from build123d import *

# Parameters (mm, degrees)
SKETCH_1_W          = 15
SKETCH_1_H          = 15
SKETCH_1_W_2        = 12
SKETCH_1_H_2        = 12
EXTRUDE_1_DEPTH     = 600
SKETCH_2_R          = 2.7
CUT_EXTRUDE_1_DEPTH = 25
SKETCH_3_R          = 2.25
CUT_EXTRUDE_2_DEPTH = 25
SKETCH_4_R          = 2.7
CUT_EXTRUDE_3_DEPTH = 20
SKETCH_5_R          = 5
CUT_EXTRUDE_4_DEPTH = 10
SKETCH_6_R          = 5
CUT_EXTRUDE_5_DEPTH = 10


with BuildPart() as part:
    # ｽｹｯﾁ1 → ﾎﾞｽ - 押し出し1 (new body)
    with BuildSketch(Plane.XY):
        Rectangle(SKETCH_1_W, SKETCH_1_H)
        Rectangle(SKETCH_1_W_2, SKETCH_1_H_2, mode=Mode.SUBTRACT)
    extrude(amount=EXTRUDE_1_DEPTH)

    # ｽｹｯﾁ2 → ｶｯﾄ - 押し出し1 (cut)
    with BuildSketch(Plane(origin=(7.5, 0, 0), x_dir=(0, 0, -1), z_dir=(1, 0, 0))):
        with Locations((-592.5, 0)):
            Circle(SKETCH_2_R)
        with Locations((-7.5, 0)):
            Circle(SKETCH_2_R)
    extrude(amount=-CUT_EXTRUDE_1_DEPTH, mode=Mode.SUBTRACT)

    # ｽｹｯﾁ3 → ｶｯﾄ - 押し出し2 (cut)
    with BuildSketch(Plane(origin=(0, 7.5, 0), x_dir=(1, 0, 0), z_dir=(0, 1, 0))):
        with Locations((0, -22.5)):
            Circle(SKETCH_3_R)
        with Locations((0, -577.5)):
            Circle(SKETCH_3_R)
        with Locations((0, -248.5)):
            Circle(SKETCH_3_R)
        with Locations((0, -351.5)):
            Circle(SKETCH_3_R)
    extrude(amount=-CUT_EXTRUDE_2_DEPTH, mode=Mode.SUBTRACT)

    # ｽｹｯﾁ4 → ｶｯﾄ - 押し出し3 (cut)
    with BuildSketch(Plane(origin=(7.5, 0, 0), x_dir=(0, 0, -1), z_dir=(1, 0, 0))):
        with Locations((-366.5, 0)):
            Circle(SKETCH_4_R)
        with Locations((-233.5, 0)):
            Circle(SKETCH_4_R)
    extrude(amount=-CUT_EXTRUDE_3_DEPTH, mode=Mode.SUBTRACT)

    # ｽｹｯﾁ5 → ｶｯﾄ - 押し出し4 (cut)
    with BuildSketch(Plane(origin=(7.5, 0, 0), x_dir=(0, 0, -1), z_dir=(1, 0, 0))):
        with Locations((-592.5, 0)):
            Circle(SKETCH_5_R)
        with Locations((-366.5, 0)):
            Circle(SKETCH_5_R)
        with Locations((-233.5, 0)):
            Circle(SKETCH_5_R)
        with Locations((-7.5, 0)):
            Circle(SKETCH_5_R)
    extrude(amount=-CUT_EXTRUDE_4_DEPTH, mode=Mode.SUBTRACT)

    # ｽｹｯﾁ6 → ｶｯﾄ - 押し出し5 (cut)
    with BuildSketch(Plane(origin=(0, -7.5, 0), x_dir=(-1, 0, 0), z_dir=(0, -1, 0))):
        with Locations((0, -577.5)):
            Circle(SKETCH_6_R)
        with Locations((0, -22.5)):
            Circle(SKETCH_6_R)
        with Locations((0, -248.5)):
            Circle(SKETCH_6_R)
        with Locations((0, -351.5)):
            Circle(SKETCH_6_R)
    extrude(amount=-CUT_EXTRUDE_5_DEPTH, mode=Mode.SUBTRACT)


solid = part.part
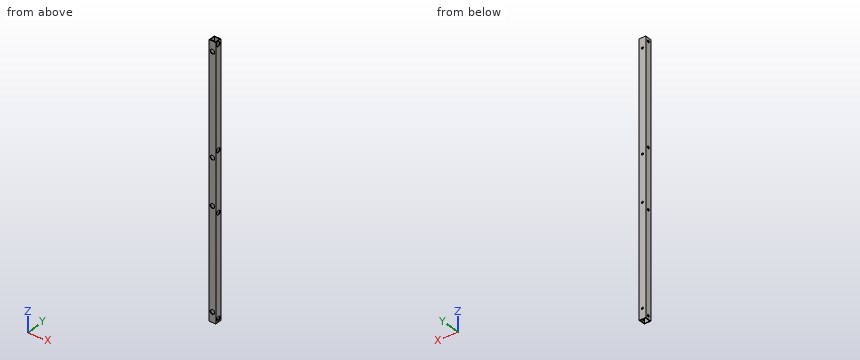
Could you check a few things on this model? Use its own coordinates, in mm. Give positions to 0.01 mm unless a question says otherwise; leave off trailing zeros. Order: outer loops, then holes, each group sorted by start corner. A loop starts at its lowest first (then second) coordinate and runs counter-clockwise, first axis right, second up. Notation, with made-up numbers: (60.25, 78) - (80.25, 78) arc R29 ccw to (80.25, 104) - close; hole circle Ø9 at (41, 54). An arc over 180 degrees is marked (long way). One line per item, written item: value. Start each with the question number.
1. For P1, Ø7, axis at y = 0, z = 592.5, coming from the +X side; P2, Ø6, axis at x = 0, z = 22.5, coming from the -Y side; P3, Ø4.5, axis at y = 0, z = 7.5, coming from the +X side, each with a flat end and sliding along its axis, tell me the tip position at first contact or that it passes through.
2. If I drill on probe 1 along Y at (x, z) = (1, 374.5); probe 2 along X at (y, z) = (-7.15, 577.5), over which ranges is the centre line in solid material (lowest first)?
3. Imagine slicing it at A-A on z = 143. List the corners of the cut face in (x, y) for me.
Values:
1. P1: x = -6
1. P2: y = 6
1. P3: through
2. probe 1: -7.5 to -6, 6 to 7.5
2. probe 2: -7.5 to -5, 5 to 7.5
3. outline: (-7.5, -7.5) - (7.5, -7.5) - (7.5, 7.5) - (-7.5, 7.5) - close; hole (-6, -6) - (6, -6) - (6, 6) - (-6, 6) - close
